```python
from build123d import *

# Parameters (mm, degrees)
SKETCH2_R           = 31
SKETCH2_R_2         = 7.5
BOSS_EXTRUDE1_DEPTH = 3


with BuildPart() as part:
    # Sketch2 → Boss-Extrude1 (new body)
    with BuildSketch(Plane(origin=(0, 0, 0), x_dir=(1, 0, 0), z_dir=(0, 1, 0))):
        Circle(SKETCH2_R)
        with Locations((0, 21.5)):
            Circle(SKETCH2_R_2, mode=Mode.SUBTRACT)
        with Locations((18.619546181, 10.75)):
            Circle(SKETCH2_R_2, mode=Mode.SUBTRACT)
        with Locations((18.619546181, -10.75)):
            Circle(SKETCH2_R_2, mode=Mode.SUBTRACT)
        with Locations((0, -21.5)):
            Circle(SKETCH2_R_2, mode=Mode.SUBTRACT)
        with Locations((-18.619546181, -10.75)):
            Circle(SKETCH2_R_2, mode=Mode.SUBTRACT)
        with Locations((-18.619546181, 10.75)):
            Circle(SKETCH2_R_2, mode=Mode.SUBTRACT)
        with BuildLine():
            Line((-2.121320344, 1.75), (2.121320344, 1.75))
            ThreePointArc((2.121320344, 1.75), (2.75, 0), (2.121320344, -1.75))
            Line((2.121320344, -1.75), (-2.121320344, -1.75))
            ThreePointArc((-2.121320344, -1.75), (-2.75, 0), (-2.121320344, 1.75))
        make_face(mode=Mode.SUBTRACT)
    extrude(amount=BOSS_EXTRUDE1_DEPTH)


solid = part.part
```
Can you work these out from the model? Positions are in its coordinate system, mm. A direction names the side the tool comes from. Give positions to 0.01 mm unless a question says otherwise; leave off trailing zeros. Loops run counter-clockwise (first coordinate to the right, second up) from the corner with the lowest first, then second, coordinate; pieces in that order, holes last. Notation, with made-up numbers: M -5,13.25 L 18,13.25 A17 ccw 18,35.25 Z; hole C 66,12 d8. An arc over 180 degrees is marked long. Answer in a Markdown table with one row per item.
1. Thinking about a two-plate mould opening in Z: for faces 3 (the flat face through (0, 3, 6)), 4 (the cylindrical face through (-24.571, 1.479, 15.314)), 5 (the cylindrical face through (-4.036, 1.479, -30.736)), which applies, released by +Z, released by -Z, zero draft, split by the parting line, or undercut?
Taken from the geometry:
| item | result |
|---|---|
| face 3 | zero draft |
| face 4 | undercut |
| face 5 | split by the parting line |
2. Suppose I cut it at C-C on y = 0.95. Write out the boundary of the cut face in (x, z), plus the area to 3 significant figures.
Taken from the geometry:
| item | result |
|---|---|
| outline | C 0,0 d62; hole C -18.62,-10.75 d15; hole C -18.62,10.75 d15; hole C 0,-21.5 d15; hole C 0,21.5 d15; hole M -2.12,-1.75 L 2.12,-1.75 A2.75 ccw 2.12,1.75 L -2.12,1.75 A2.75 ccw Z; hole C 18.62,-10.75 d15; hole C 18.62,10.75 d15 |
| area | 1,940 mm² |
3. Suppose I cut it at D-D on x = 14. Write out the boundary of the cut face in (y, z).
Taken from the geometry:
| item | result |
|---|---|
| outline | M 0,-27.66 L 3,-27.66 L 3,-16.66 L 0,-16.66 Z; M 0,-4.84 L 3,-4.84 L 3,4.84 L 0,4.84 Z; M 0,16.66 L 3,16.66 L 3,27.66 L 0,27.66 Z |
4. Suppose I cut it at B-B on x = 0. Write out the boundary of the cut face in (y, z), plus the area to 3 significant figures.
Taken from the geometry:
| item | result |
|---|---|
| outline | M 0,-31 L 3,-31 L 3,-29 L 0,-29 Z; M 0,-14 L 3,-14 L 3,-1.75 L 0,-1.75 Z; M 0,1.75 L 3,1.75 L 3,14 L 0,14 Z; M 0,29 L 3,29 L 3,31 L 0,31 Z |
| area | 85.5 mm² |
5. If I drill on line 1 along Z through (x, y) = (0, 0.9); line 2 along Z through (x, y) = (19, 0.65); line 3 along Z through (x, y) = (14.5, 0.2), over which ranges is the centre line in solid material (lowest first)?
Taken from the geometry:
| item | result |
|---|---|
| line 1 | z = -31 to -29, -14 to -1.75, 1.75 to 14, 29 to 31 |
| line 2 | z = -24.49 to -18.24, -3.26 to 3.26, 18.24 to 24.49 |
| line 3 | z = -27.4 to -17.02, -4.48 to 4.48, 17.02 to 27.4 |
6. For pin 1 Ø13.5 at (x, z) = (-18.62, 10.75) entering from +Y; pin 2 Ø0.9 at (x, y) = (0.5, 2) entering from +Z; pin 3 Ø19.5 at (x, z) = (18.62, -10.75) entering from +Y; pin 4 Ø1.5 at (x, y) = (-14, 1) entering from +Z, each with a flat end and sliding along its axis, tell me the tip position at first contact or that it passes through.
Taken from the geometry:
| item | result |
|---|---|
| pin 1 | passes through |
| pin 2 | stops at z = 31 |
| pin 3 | stops at y = 3 |
| pin 4 | stops at z = 28.03 |
7. Suppose I cut it at A-A on z = 0. Write out the boundary of the cut face in (x, y).
Taken from the geometry:
| item | result |
|---|---|
| outline | M -31,0 L -2.75,0 L -2.75,3 L -31,3 Z; M 2.75,0 L 31,0 L 31,3 L 2.75,3 Z |
8. Which directions (+Z, -Z, +X, -X, +Y, -Y) give clear straight access to the entire face, cutting with the end or side of a thin tool? Please do faces 1 (the cylindrical face through (2.75, 1.48, -0.03)), 2 (the flat face through (0, 0, 6)).
Taken from the geometry:
| item | result |
|---|---|
| face 1 | +Y, -Y |
| face 2 | +Z, -Z, +X, -X, -Y |
